Build history of the part. All positions in model axes, mm. Face numbers are marked on the shaded views. A direction names the side the tool comes from. Give positions to 0.01 mm unless a question says otherwise; leave off trailing zeros. Write each loop counter-clockwise with the first axis right and the second up, starting at its lowest first coordinate (ties: lowest second). Pieces come first, ordered by that corner, then holes. Notation, with made-up numbers: M 48.5,4 L 87.5,4 A34 ccw 87.5,39 Z; hole C 29.25,-31.75 d5. An arc over 180 degrees is marked long. Return JSON: item names as keys, results as strings. Group by question number.
Q1. Band-saw the part on A-A, the plane z = -38.1. Give the cut face in (x, y) (1 decimal).
Q2. Band-saw the part on B-B, the plane x = 12.5. Give the cut face in (y, z) (3 decimals).
Q3. Band-saw the part on C-C, the plane y = 130.5. Give the cut face in (x, z) (3 decimals), then the cut area to 3 significant figures.
Q4. Pull direction X, two halves, no side cores. Call the marked faces 5, 6 and 7: +X half, -X half, draft (parallel to the pull), parting line (faces both ways), or undercut.
Q5. Tool access for the marked faces 1, 2, 3 and 4: list every direction of +Z, -Z, +X, -X, +Y, -Y with a clear straight run to the whole face (end or side of a thin tool).
Q6. Flat gauge pins, fed straight in: pin 1 Ø10 at (y, z) = (104.5, 11) entering from +X; pin 2 Ø8 at (y, z) = (69.5, 25.5) entering from +X; pin 3 Ø6.5 at (x, z) = (2.5, -24.5) entering from -Y; pin 4 Ø5 at (y, z) = (120, -14.5) entering from -X. Where does each tip first touch, or does it go through?
Q7. Wall check: probe 1 along Z at (x, y) = (0, 34.75) (1 decimal); probe 2 along Y at (x, z) = (-2, 28.5); probe 3 along X at (y, z) = (20.25, -38.1) (1 decimal). Give the ranges that are in metal, low to high.
Q8. Band-saw the part on D-D, the plane z = 3. Give the cut face in (x, y) (3 decimals).
from build123d import *

# Parameters (mm, degrees)
CUT_EXTRUDE1_DEPTH      = 120.65
CUT_EXTRUDE2_DEPTH      = 107.95
CUT_EXTRUDE3_DEPTH      = 167.225729431
CUT_EXTRUDE3_DEPTH_BACK = 167.225729431
SKETCH5_R               = 4.7625
CUT_EXTRUDE4_DEPTH      = 139.176350183


with BuildPart() as part:
    # Sketch1 → Revolve1 (revolve)
    with BuildSketch(Plane(origin=(0, 0, 0), x_dir=(0, 0, -1), z_dir=(1, 0, 0))):
        Polygon((0, 0), (47.625, 0), (47.625, 146.05), (0, 146.05), (0, 38.1), (7.9375, 38.1), (7.9375, 28.575), (0, 28.575), align=None)
    revolve(axis=Axis((0, 0, 0), (0, 1, 0)))

    # Sketch2 → Cut-Extrude1 (cut)
    with BuildSketch(Plane(origin=(0, 146.05, 0), x_dir=(1, 0, 0), z_dir=(0, 1, 0))):
        with BuildLine():
            ThreePointArc((38.1, 28.575), (0, 47.625), (-38.1, 28.575))
            Line((-38.1, 28.575), (38.1, 28.575))
        make_face()
        with BuildLine():
            Line((38.1, -28.575), (-38.1, -28.575))
            ThreePointArc((-38.1, -28.575), (0, -47.625), (38.1, -28.575))
        make_face()
    extrude(amount=-CUT_EXTRUDE1_DEPTH, mode=Mode.SUBTRACT)

    # Sketch2<3> → Cut-Extrude2 (cut)
    with BuildSketch(Plane(origin=(0, 146.05, 0), x_dir=(1, 0, 0), z_dir=(0, 1, 0))):
        with BuildLine():
            ThreePointArc((-44.901280605, 15.875), (-46.939131403, 8.053481737), (-47.625, 0))
            Line((-47.625, 0), (47.625, 0))
            ThreePointArc((47.625, 0), (46.939131403, 8.053481737), (44.901280605, 15.875))
            Line((44.901280605, 15.875), (-44.901280605, 15.875))
        make_face()
        with BuildLine():
            Line((47.625, 0), (-47.625, 0))
            ThreePointArc((-47.625, 0), (-46.939131403, -8.053481737), (-44.901280605, -15.875))
            Line((-44.901280605, -15.875), (44.901280605, -15.875))
            ThreePointArc((44.901280605, -15.875), (46.939131403, -8.053481737), (47.625, 0))
        make_face()
    extrude(amount=-CUT_EXTRUDE2_DEPTH, mode=Mode.SUBTRACT)

    # Sketch4 → Cut-Extrude3 (cut, two sides)
    with BuildSketch(Plane.XY.offset(-15.875)) as cut_extrude3_sk:
        with BuildLine():
            Line((-28.575, 57.498647721), (-28.575, 38.1))
            Line((-28.575, 38.1), (0, 38.1))
            Line((0, 38.1), (0, 107.95))
            Line((0, 107.95), (-9.412473661, 107.95))
            ThreePointArc((-9.412473661, 107.95), (-13.158337818, 106.72747518), (-15.461867516, 103.530630463))
            Line((-15.461867516, 103.530630463), (-27.071969275, 67.151800038))
            ThreePointArc((-27.071969275, 67.151800038), (-28.196992083, 62.38338034), (-28.575, 57.498647721))
        make_face()
        with BuildLine():
            Line((0, 107.95), (0, 38.1))
            Line((0, 38.1), (28.575, 38.1))
            Line((28.575, 38.1), (28.575, 57.498647721))
            ThreePointArc((28.575, 57.498647721), (28.196992083, 62.38338034), (27.071969275, 67.151800038))
            Line((27.071969275, 67.151800038), (15.461867516, 103.530630463))
            ThreePointArc((15.461867516, 103.530630463), (13.158337818, 106.72747518), (9.412473661, 107.95))
            Line((9.412473661, 107.95), (0, 107.95))
        make_face()
        with BuildLine():
            Line((-44.901280605, 146.05), (-44.901280605, 63.5))
            Line((-44.901280605, 63.5), (-24.19757542, 128.372521853))
            ThreePointArc((-24.19757542, 128.372521853), (-14.983456626, 141.15990072), (0, 146.05))
            Line((0, 146.05), (-44.901280605, 146.05))
        make_face()
        with BuildLine():
            Line((44.901280605, 146.05), (0, 146.05))
            ThreePointArc((0, 146.05), (14.983456626, 141.15990072), (24.19757542, 128.372521853))
            Line((24.19757542, 128.372521853), (44.901280605, 63.5))
            Line((44.901280605, 63.5), (44.901280605, 146.05))
        make_face()
        with BuildLine():
            ThreePointArc((5.55625, 120.65), (3.928862053, 124.578862053), (0, 126.20625))
            Line((0, 126.20625), (0, 115.09375))
            ThreePointArc((0, 115.09375), (3.928862053, 116.721137947), (5.55625, 120.65))
        make_face()
        with BuildLine():
            Line((0, 115.09375), (0, 126.20625))
            ThreePointArc((0, 126.20625), (-5.55625, 120.65), (0, 115.09375))
        make_face()
    extrude(amount=CUT_EXTRUDE3_DEPTH, mode=Mode.SUBTRACT)
    extrude(cut_extrude3_sk.sketch, amount=-CUT_EXTRUDE3_DEPTH_BACK, mode=Mode.SUBTRACT)

    # Sketch5 → Cut-Extrude4 (cut, through all)
    with BuildSketch(Plane(origin=(0, 25.4, 0), x_dir=(1, 0, 0), z_dir=(0, 1, 0))):
        with Locations(Location((0, -38.1, 0), (0, 0, 270))):
            Circle(SKETCH5_R)
        with Locations(Location((0, 38.1, 0), (0, 0, 90))):
            Circle(SKETCH5_R)
    extrude(amount=-CUT_EXTRUDE4_DEPTH, mode=Mode.SUBTRACT)


solid = part.part
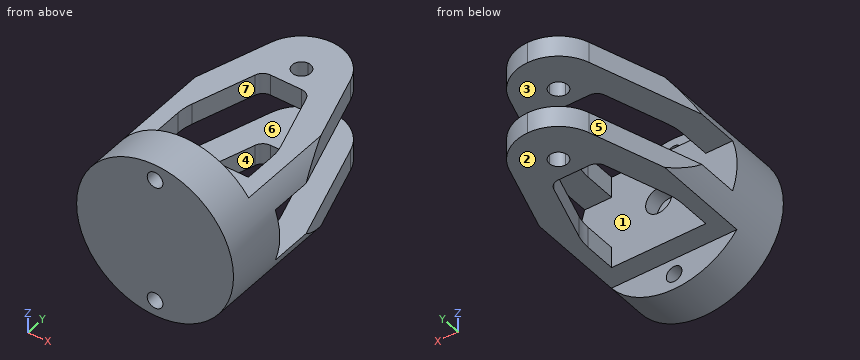
From the geometry:
{
 "1": {"outline": "M -28.6,0 L -4.8,0 L -4.8,25.4 L -28.6,25.4 Z; M 4.8,0 L 28.6,0 L 28.6,25.4 L 4.8,25.4 Z"},
 "2": {"outline": "M 0,-45.955 L 25.4,-45.955 L 25.4,-28.575 L 38.1,-28.575 L 38.1,28.575 L 25.4,28.575 L 25.4,45.955 L 0,45.955 Z; M 107.149,-28.575 L 142.761,-28.575 L 142.761,-15.875 L 107.149,-15.875 Z; M 107.149,15.875 L 142.761,15.875 L 142.761,28.575 L 107.149,28.575 Z"},
 "3": {"outline": "M -23.412,-28.575 L 23.412,-28.575 L 23.412,-15.875 L -23.412,-15.875 Z; M -23.412,15.875 L 23.412,15.875 L 23.412,28.575 L -23.412,28.575 Z", "area": "1,190 mm^2"},
 "4": {"face 5": "-X half", "face 6": "draft", "face 7": "undercut"},
 "5": {"face 1": "none", "face 2": "-Z, +X, -X, +Y", "face 3": "+X, -X, +Y", "face 4": "+Z, -Z"},
 "6": {"pin 1": "stops at x = 32.17", "pin 2": "stops at x = 42.5", "pin 3": "stops at y = 0", "pin 4": "stops at x = -27.54"},
 "7": {"probe 1": "z = -28.6 to -7.9, 7.9 to 28.6", "probe 2": "y = 0 to 38.1, 107.95 to 115.47, 125.83 to 145.97", "probe 3": "x = -28.6 to -4.8, 4.8 to 28.6"},
 "8": {"outline": "M -47.53,0 L 47.53,0 L 47.53,38.1 L 7.349,38.1 L 7.349,28.575 L -7.349,28.575 L -7.349,38.1 L -47.53,38.1 Z"}
}
